Design review of the part shown in the three views and the two pictorial views. Dimensions are in mm from the part's minimum x, y and z. Give positions to 0.01 mm unless a question says otherwise; leave off trailing zeros. Order: outer loops, then holes, each group sorted by start corner. A loop starts at its lowest first (then second) coordinate and runs counter-clockwise, first axis right, second up.
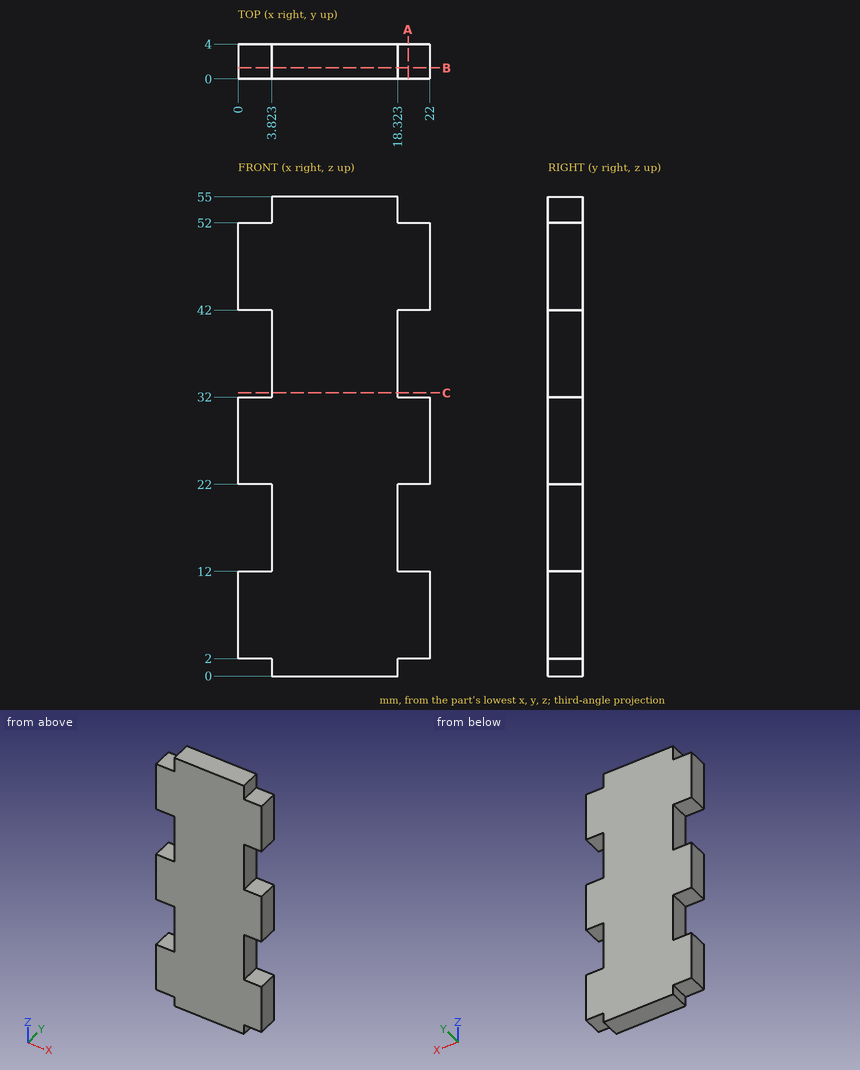
Item 1: Take a section at B-B (y = 1.25). Give the boundary of the cut face in (x, z).
Values found:
outline: (0, 2) - (3.82, 2) - (3.82, 0) - (18.32, 0) - (18.32, 2) - (22, 2) - (22, 12) - (18.32, 12) - (18.32, 22) - (22, 22) - (22, 32) - (18.32, 32) - (18.32, 42) - (22, 42) - (22, 52) - (18.32, 52) - (18.32, 55) - (3.82, 55) - (3.82, 52) - (0, 52) - (0, 42) - (3.82, 42) - (3.82, 32) - (0, 32) - (0, 22) - (3.82, 22) - (3.82, 12) - (0, 12) - close
Item 2: Clearance check with flat-ended pins moving along their axes: pin 1 Ø1.1 at (x, y) = (20, 1.5) entering from +Z; pin 2 Ø0.6 at (y, z) = (2, 1.5) entering from +X; pin 3 Ø1 at (y, z) = (1, 0.5) entering from -X. State where each tip first meets the part, or that it passes through.
Values found:
pin 1: stops at z = 52
pin 2: stops at x = 18.32
pin 3: stops at x = 3.82
Item 3: For line 1 (Z direction, x = 19, y = 2); line 2 (X direction, y = 0.2, z = 14), list the stretches that pass through material, from the lowest coordinate up.
Values found:
line 1: z = 2 to 12, 22 to 32, 42 to 52
line 2: x = 3.82 to 18.32
Item 4: Take a section at A-A (x = 19.5). Give the boundary of the cut face in (y, z).
Values found:
outline: (0, 2) - (4, 2) - (4, 12) - (0, 12) - close; (0, 22) - (4, 22) - (4, 32) - (0, 32) - close; (0, 42) - (4, 42) - (4, 52) - (0, 52) - close
Item 5: Take a section at C-C (z = 32.5). Give the boundary of the cut face in (x, y), and give its area (3 significant figures).
Values found:
outline: (3.82, 0) - (18.32, 0) - (18.32, 4) - (3.82, 4) - close
area: 58.0 mm2
